Read the model definition and answer for the solid it produces. Units are mm, in the model's axes. Round coordinates to 2 decimals unless told otherwise and drop trailing zeros. Write each loop counter-clockwise with the first axis right and the second up, starting at its lowest first coordinate (ties: lowest second). Pieces come first, ordered by that corner, then holes. Notation, with made-up numbers: M 16,62 L 48,62 A8 ccw 48,73 Z; hole C 50.25,81.25 d3. An arc over 180 degrees is marked long. Use one line per item in the form item = value. Start each with the question number.
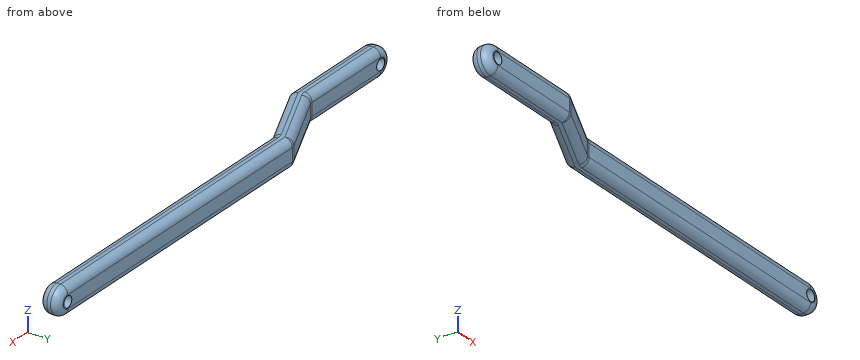
```python
from build123d import *

# Parameters (mm, degrees)
CROQUIS1_R                 = 3
SALIENTE_EXTRUIR1_DEPTH    = 13.75
CORTAR_EXTRUIR1_DEPTH      = 268.958135723
CORTAR_EXTRUIR1_DEPTH_BACK = 268.958135723
CROQUIS3_OUTSIDE_W         = 84.856
CROQUIS3_OUTSIDE_H         = 332.356
REDONDEO5_R                = 4


with BuildPart() as part:
    # Croquis1 → Saliente-Extruir1 (new, symmetric)
    with BuildSketch(Plane(origin=(0, 0, 0), x_dir=(-1, 0, 0), z_dir=(0, 1, 0))):
        with BuildLine():
            Line((0, 7.5), (260, 7.5))
            ThreePointArc((260, 7.5), (267.5, 0), (260, -7.5))
            Line((260, -7.5), (0, -7.5))
            ThreePointArc((0, -7.5), (-7.5, 0), (0, 7.5))
        make_face()
        with Locations(Location((0, 0, 0), (0, 0, 90))):
            Circle(CROQUIS1_R, mode=Mode.SUBTRACT)
        with Locations(Location((260, 0, 0), (0, 0, 90))):
            Circle(CROQUIS1_R, mode=Mode.SUBTRACT)
    extrude(amount=SALIENTE_EXTRUIR1_DEPTH, both=True)

    # Croquis3 outside → Cortar-Extruir1 (cut, two sides: drawn at the far end of the back side and taken through both)
    with BuildSketch(Plane(origin=(0, 0, 0), x_dir=(0, 1, 0), z_dir=(0, 0, 1)).offset(-CORTAR_EXTRUIR1_DEPTH_BACK)):
        with Locations((0, 130)):
            Rectangle(CROQUIS3_OUTSIDE_W, CROQUIS3_OUTSIDE_H)
        Polygon((13.75, 169.971128891), (13.75, -7.5), (3.75, -7.5), (3.75, 167.754182265), (-13.75, 205.283053374), (-13.75, 267.5), (-3.75, 267.5), (-3.75, 207.5), align=None, mode=Mode.SUBTRACT)
    extrude(amount=CORTAR_EXTRUIR1_DEPTH + CORTAR_EXTRUIR1_DEPTH_BACK, mode=Mode.SUBTRACT)

    # Redondeo5
    redondeo5_edges = [part.edges().sort_by_distance(p)[0] for p in [
        (-84.985564446, 13.75, 7.5),
        (-232.641526687, -13.75, -7.5),
        (-186.518617819, -5, -7.5),
        (-83.877091132, 3.75, -7.5),
        (-167.754182265, 3.75, 0),
        (-83.877091132, 3.75, 7.5),
        (7.5, 3.75, 0),
        (-207.5, -3.75, 0),
        (-233.75, -3.75, 7.5),
        (-267.5, -3.75, 0),
        (-188.735564446, 5, -7.5),
        (-233.75, -3.75, -7.5),
        (-169.971128891, 13.75, 0),
        (-188.735564446, 5, 7.5),
        (-205.283053374, -13.75, 0),
        (-186.518617819, -5, 7.5),
        (7.5, 13.75, 0),
        (-232.641526687, -13.75, 7.5),
        (-267.5, -13.75, 0),
        (-84.985564446, 13.75, -7.5),
    ]]
    fillet(redondeo5_edges, radius=REDONDEO5_R)


solid = part.part
```
Q1. Find section B-B on z = 0. Count the separate pieces of the cut face and the enclosed holes in it, and give its area (3 significant figures).
Q2. Find section A-A on x = -231. Write down the section's boundary in (y, z).
Q3. Each of these flat-tipped pins is pushed along its axis until it touches: pin 1 Ø2 at (x, z) = (-80, 0.5) entering from -Y; pin 2 Ø5 at (y, z) = (-3.5, -0.5) entering from +X; pin 3 Ø5.5 at (x, z) = (-234, -1) entering from +Y. Where does it stop, or does it pass through?
Q4. Straight lines are drawn through the part: line 1 (Z direction, x = -260, y = -9.5); line 2 (Y direction, x = -245, z = 2.5); line 3 (Y direction, x = -9.5, z = -3.25). For each, find the intervals that lie inside material, in ascending order. Write a range as [from, to].
Response:
q1.separate_pieces = 3
q1.enclosed_holes = 0
q1.area = 2,660 mm²
q2.outline = M -13.75,-3.5 A4 ccw -9.75,-7.5 L -7.75,-7.5 A4 ccw -3.75,-3.5 L -3.75,3.5 A4 ccw -7.75,7.5 L -9.75,7.5 A4 ccw -13.75,3.5 Z
q3.pin_1 = 3.75
q3.pin_2 = -177.94
q3.pin_3 = -3.75
q4.line_1 = [-7.5, -3], [3, 7.5]
q4.line_2 = [-13.75, -3.75]
q4.line_3 = [3.75, 13.75]
